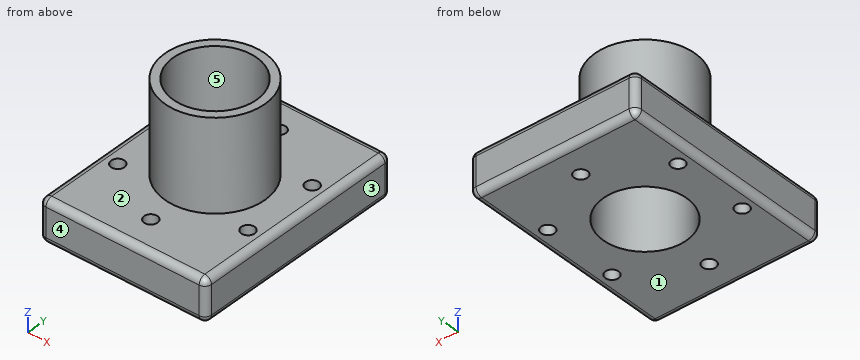
```python
from build123d import *

# Parameters (mm, degrees)
F0_W     = 50
F0_H     = 65
F0_R     = 2
F0_R_2   = 15
F1_DEPTH = 12.7
F2_R     = 2
F0_R_3   = 12.5
F3_DEPTH = 40


with BuildPart() as f1:
    # F0 (on Top) → F1 (new body)
    with BuildSketch(Plane.XY):
        Rectangle(F0_W, F0_H)
        with Locations((-19.55572, -11.2905)):
            Circle(F0_R, mode=Mode.SUBTRACT)
        with Locations((0, -22.581)):
            Circle(F0_R, mode=Mode.SUBTRACT)
        with Locations((19.55572, -11.2905)):
            Circle(F0_R, mode=Mode.SUBTRACT)
        with Locations((-19.55572, 11.2905)):
            Circle(F0_R, mode=Mode.SUBTRACT)
        Circle(F0_R_2, mode=Mode.SUBTRACT)
        with Locations((19.55572, 11.2905)):
            Circle(F0_R, mode=Mode.SUBTRACT)
        with Locations((0, 22.581)):
            Circle(F0_R, mode=Mode.SUBTRACT)
    extrude(amount=F1_DEPTH)

    # F2
    f2_edges = [f1.edges().sort_by_distance(p)[0] for p in [
        (-25, 32.5, 6.35),
        (-25, -32.5, 6.35),
        (-25, 0, 0),
        (-25, 0, 12.7),
        (25, -32.5, 6.35),
        (0, -32.5, 0),
        (0, -32.5, 12.7),
        (25, 32.5, 6.35),
        (25, 0, 0),
        (25, 0, 12.7),
        (0, 32.5, 0),
        (0, 32.5, 12.7),
    ]]
    fillet(f2_edges, radius=F2_R)

    # F0 (on Top) → F3 (join)
    with BuildSketch(Plane.XY):
        Circle(F0_R_2)
        Circle(F0_R_3, mode=Mode.SUBTRACT)
    extrude(amount=F3_DEPTH)


solid = f1.part
```
Can you work these out from the model? Positions are in its coordinate system, mm. Face numbers are marked on the shaded views. A direction names the side the tool comes from. Give positions to 0.01 mm unless a question says otherwise; leave off trailing zeros. Order: outer loops, then holes, each group sorted by start corner. A loop starts at its lowest first (then second) coordinate and runs counter-clockwise, first axis right, second up. Notation, with made-up numbers: (-16.75, 35.5) - (-12.75, 35.5) arc R17 cw to (-12.75, 51.5) - close; hole circle Ø1 at (6.5, 45). An arc over 180 degrees is marked (long way). Use a Markdown table: item, result. Add a question column.
Q1. If we section it at B-B on x = 20: Write out the boundary of the cut face in (y, z), plus the area to 3 significant figures.
Q2. If we section it at A-A on y = 0: Write out the boundary of the cut face in (x, z), plus the area to 3 significant figures.
Q3. On a 3-axis mill with a long thin cutter (end or side, diameter ignored), from which of +Z, -Z, +X, -X, +Y, -Y can I reach the whole of each face in a straight line? I mean the marked faces 1 and 2. Say none if no direction works.
Q4. If we section it at C-C on x = 0: Write out the boundary of the cut face in (y, z).
Q5. If we mould it in two halves opening along Y, with no side actions, what happens to the marked faces 3, 4 and 5? For each: released by +Y, released by -Y, zero draft, split by the parting line, or undercut.
Q6. If we section it at D-D on y = -19: Write out the boundary of the cut face in (x, z), plus the area to 3 significant figures.
Q7. I'm going to push flat-ended pins straight in: pin 1 (12 mm diameter, centred on x = -18.5, y = 9, fed in from -Z); pin 2 (1.5 mm diameter, centred on y = 11.5, z = 33.5, fed in from -X); pin 3 (5 mm diameter, centred on x = 19.56, y = 11.29, fed in from +Z); pin 4 (10 mm diameter, centred on x = 10.5, z = 16, fed in from +Y). Where does each tip first touch, or does it pass through?
Q8. Please list where these lines run through material, in increasing order: line 1 along Y through (x, z) = (21, 12.5); line 2 along Y through (x, z) = (0, 24); line 3 along X through (y, z) = (13, 9.5).
Answers follow:
| question | item | result |
|---|---|---|
| 1 | outline | (-32.5, 2) arc R2 ccw to (-30.5, 0) - (-13.24, 0) - (-13.24, 12.7) - (-30.5, 12.7) arc R2 ccw to (-32.5, 10.7) - close; (-9.34, 0) - (9.34, 0) - (9.34, 12.7) - (-9.34, 12.7) - close; (13.24, 0) - (30.5, 0) arc R2 ccw to (32.5, 2) - (32.5, 10.7) arc R2 ccw to (30.5, 12.7) - (13.24, 12.7) - close |
| 1 | area | 723 mm^2 |
| 2 | outline | (-25, 2) arc R2 ccw to (-23, 0) - (-12.5, 0) - (-12.5, 40) - (-15, 40) - (-15, 12.7) - (-23, 12.7) arc R2 ccw to (-25, 10.7) - close; (12.5, 0) - (23, 0) arc R2 ccw to (25, 2) - (25, 10.7) arc R2 ccw to (23, 12.7) - (15, 12.7) - (15, 40) - (12.5, 40) - close |
| 2 | area | 451 mm^2 |
| 3 | face 1 | -Z, +X, -X, +Y, -Y |
| 3 | face 2 | +Z |
| 4 | outline | (-32.5, 2) arc R2 ccw to (-30.5, 0) - (-24.58, 0) - (-24.58, 12.7) - (-30.5, 12.7) arc R2 ccw to (-32.5, 10.7) - close; (-20.58, 0) - (-12.5, 0) - (-12.5, 40) - (-15, 40) - (-15, 12.7) - (-20.58, 12.7) - close; (12.5, 0) - (20.58, 0) - (20.58, 12.7) - (15, 12.7) - (15, 40) - (12.5, 40) - close; (24.58, 0) - (30.5, 0) arc R2 ccw to (32.5, 2) - (32.5, 10.7) arc R2 ccw to (30.5, 12.7) - (24.58, 12.7) - close |
| 5 | face 3 | zero draft |
| 5 | face 4 | released by -Y |
| 5 | face 5 | undercut |
| 6 | outline | (-25, 2) arc R2 ccw to (-23, 0) - (23, 0) arc R2 ccw to (25, 2) - (25, 10.7) arc R2 ccw to (23, 12.7) - (-23, 12.7) arc R2 ccw to (-25, 10.7) - close |
| 6 | area | 632 mm^2 |
| 7 | pin 1 | stops at z = 0 |
| 7 | pin 2 | stops at x = -10.46 |
| 7 | pin 3 | stops at z = 12.7 |
| 7 | pin 4 | stops at y = 32.48 |
| 8 | line 1 | y = -31.37 to -12.67, -9.91 to 9.91, 12.67 to 31.37 |
| 8 | line 2 | y = -15 to -12.5, 12.5 to 15 |
| 8 | line 3 | x = -25 to -20.59, -18.52 to 18.52, 20.59 to 25 |
